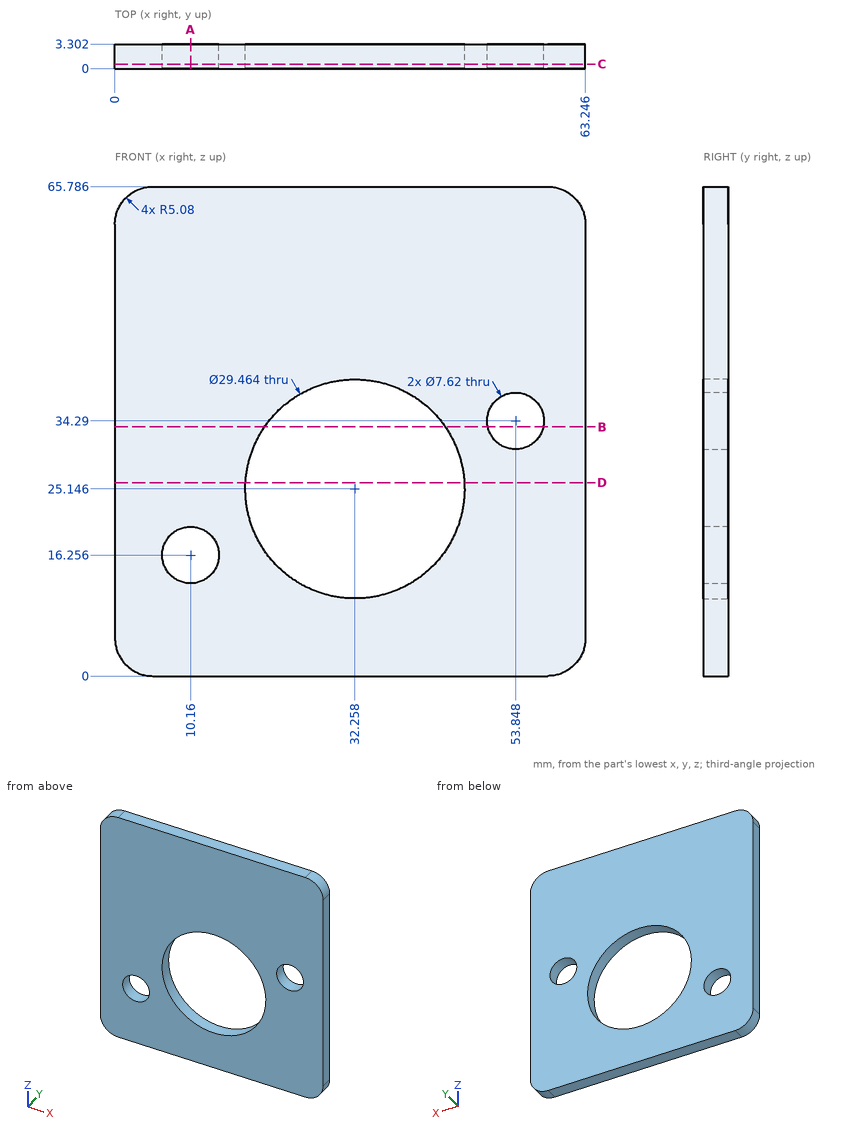
Print and shaded views of the part. All mm, measured from the part's lowest x, y and z. Round coordinates to 2 decimals unless told otherwise and drop trailing zeros. Write each loop counter-clockwise with the first axis right and the second up, starting at its lowest first coordinate (ties: lowest second). Pieces come first, ordered by that corner, then holes.
Item 1: Cut at B-B, the plane z = 33.5. Give the cut face in (x, y).
Results:
outline: (0, 0) - (20.12, 0) - (20.12, 3.3) - (0, 3.3) - close; (44.39, 0) - (50.12, 0) - (50.12, 3.3) - (44.39, 3.3) - close; (57.58, 0) - (63.25, 0) - (63.25, 3.3) - (57.58, 3.3) - close
Item 2: Cut at A-A, the plane x = 10.16. Give the cut face in (y, z).
Results:
outline: (0, 0) - (3.3, 0) - (3.3, 12.45) - (0, 12.45) - close; (0, 20.07) - (3.3, 20.07) - (3.3, 65.79) - (0, 65.79) - close
Item 3: Cut at C-C, the plane y = 0.6. Give the cut face in (x, z), plus the area to 3 significant figures.
Results:
outline: (0, 5.08) arc R5.08 ccw to (5.08, 0) - (58.17, 0) arc R5.08 ccw to (63.25, 5.08) - (63.25, 60.71) arc R5.08 ccw to (58.17, 65.79) - (5.08, 65.79) arc R5.08 ccw to (0, 60.71) - close; hole circle Ø7.62 at (10.16, 16.26); hole circle Ø29.46 at (32.26, 25.15); hole circle Ø7.62 at (53.85, 34.29)
area: 3,370 mm2
Item 4: Cut at D-D, the plane z = 26. Give the cut face in (x, y), plus the area to 3 significant figures.
Results:
outline: (0, 0) - (17.55, 0) - (17.55, 3.3) - (0, 3.3) - close; (46.97, 0) - (63.25, 0) - (63.25, 3.3) - (46.97, 3.3) - close
area: 112 mm2
Item 5: Probe L1, parallel to X at y = 2.75, z = 14; L2, parallel to X at y = 0.25, z = 25; L3, parallel to X at y = 0.7, z = 34.29. List the from-to ranges inside material, lowest first.
Results:
L1: x = 0 to 7.09, 13.23 to 22.62, 41.89 to 63.25
L2: x = 0 to 17.53, 46.99 to 63.25
L3: x = 0 to 20.71, 43.81 to 50.04, 57.66 to 63.25
